Design review of the part built by this model. Coordinates are the model's own, in mm. Face numbers are marked on the shaded views. A direction names the side the tool comes from. Give positions to 0.01 mm unless a question says otherwise; leave off trailing zeros. Order: outer loops, then holes, each group sorted by start corner. A loop starts at its lowest first (then second) coordinate and runs counter-clockwise, first axis right, second up.
```python
from build123d import *

# Parameters (mm, degrees)
F1_DEPTH = 66.675
F3_DEPTH = 234.951


with BuildPart() as f1:
    # F0 (on Right) → F1 (new body)
    with BuildSketch(Plane.YZ):
        Polygon((0, 128.5875), (0, 0), (3.175, 0), (3.175, 125.4125), (19.05, 125.4125), (19.05, 234.95), (-6.35, 234.95), (-6.35, 231.775), (15.875, 231.775), (15.875, 128.5875), align=None)
    extrude(amount=F1_DEPTH)

    # F2 (on face) → F3 (cut, through all)
    with BuildSketch(Plane.XY.offset(234.95)):
        Polygon((66.675, -6.35), (66.675, 19.05), (41.275, -6.35), align=None)
    extrude(amount=-F3_DEPTH, mode=Mode.SUBTRACT)

    # F4: F1 across face


with BuildPart() as f1_1:
    add(f1.part)
    add(f1.part.mirror(Plane(origin=(56.208576, 8.583576, 127.461483), x_dir=(0.707107, 0.707107, 0), z_dir=(0.707107, -0.707107, 0))))


solid = f1_1.part
```
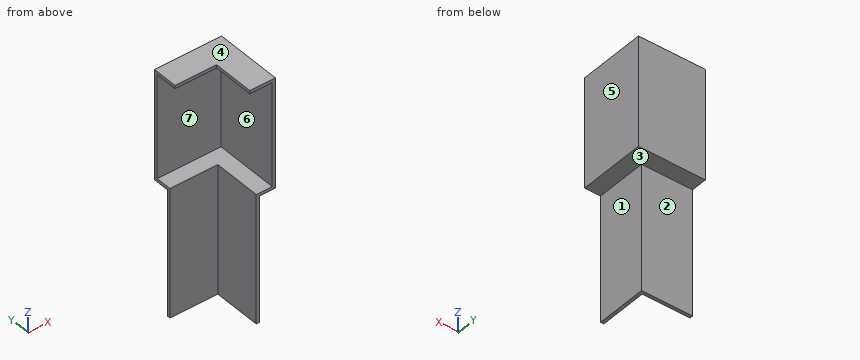
1. Take a section at C-C (z = 221.5). State the section outline as (x, y) points (3 decimals).
Recorded:
outline: (0, 15.875) - (63.5, 15.875) - (63.5, -47.625) - (66.675, -47.625) - (66.675, 19.05) - (0, 19.05) - close
2. For line 1 along Y through (x, z) = (42.5, 169) (3 decimals); line 2 along Z through (x, y) = (19.5, -5) (3 decimals); line 3 along Y through (x, z) = (7, 59) (3 decimals), list the stretches that pass through material, from the lowest coordinate up.
Recorded:
line 1: y = 15.875 to 19.05
line 2: z = 231.775 to 234.95
line 3: y = 0 to 3.175
3. Machinability: for the marked faces 1, 2 and 3, which of the approach directions +Z, -Z, +X, -X, +Y, -Y give a long, thin tool a straight path to every point of the face, cutting with its end or side? Answer none if there is none.
Recorded:
face 1: -Z, +X, +Y, -Y
face 2: -Z, +X, -X, +Y
face 3: -Z, +X, +Y
4. For pin 1 (2.5 mm diameter, centred on y = -36, z = 232.5, fed in from -X) (3 decimals); pin 2 (5 mm diameter, centred on x = 13, z = 67.5, fed in from +Y) (3 decimals); pin 3 (24 mm diameter, centred on x = 21.5, z = 39, fed in from -Y); pin 4 (5 mm diameter, centred on x = 38.5, y = -21, fed in from +Z), all flat-tipped, find the tip position at first contact; note any pin that passes through.
Recorded:
pin 1: stops at x = 41.275
pin 2: stops at y = 3.175
pin 3: stops at y = 0
pin 4: passes through
5. Draft analysis for pull direction Z (two halves, no side actions). For the marked faces 4, 5, 6 and 7, state which applies: pulls with the +Z half, pulls with the -Z half, needs draft (parallel to the pull), parting line crosses it, or undercut.
Recorded:
face 4: pulls with the +Z half
face 5: needs draft
face 6: undercut
face 7: undercut
